Read the model definition and answer for the solid it produces. Units are mm, in the model's axes. Coordinates: 2 decimals unless noted, no trailing zeros. Write each loop counter-clockwise with the first axis right and the second up, starting at its lowest first coordinate (ties: lowest second). Pieces come first, ordered by that corner, then holes.
Item 1: Section B-B (y = 2.85) is taken. Give the vertices of the cut face in (x, z).
Item 2: Section C-C (y = -0.35) is taken. Give the vertices of the cut face in (x, z).
Item 3: Straight lines are drawn through the part: probe 1 along Y at (x, z) = (34.05, 12.5); probe 2 along X at (y, z) = (2.2, 0.25); probe 3 along Y at (x, z) = (35.7, 5.75). For each, find the intervals that lie inside material, in ascending order.
Item 4: Each of these flat-tipped pins is pushed along its axis until it touches: P1, Ø1, axis at x = 33.5, z = -7.5, coming from the +Y side; P2, Ø1.5, axis at x = 34, z = -13, coming from the -Y side; P3, Ø0.9, axis at x = 34.5, y = 0, coming from the -Z side. Where does it stop, or does it pass through?
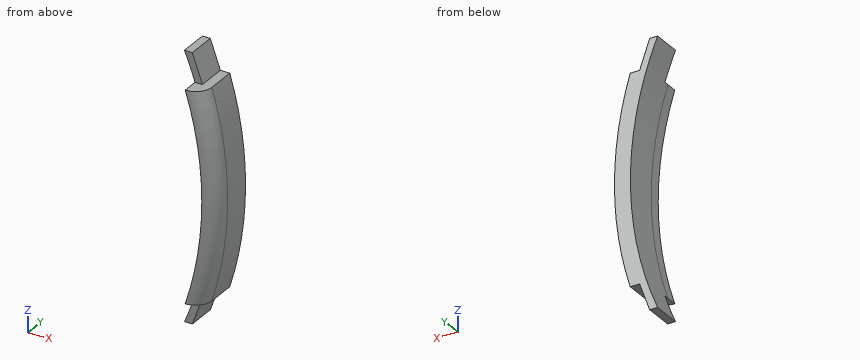
from build123d import *

# Parameters (mm, degrees)
BOSS_EXTRUDE1_DEPTH = 3.6
BOSS_EXTRUDE2_START = 1.2
BOSS_EXTRUDE2_DEPTH = 1.2
FILLET1_R           = 1.7
CUT_EXTRUDE1_DEPTH  = 0.5


with BuildPart() as part:
    # Sketch1 → Boss-Extrude1 (new body)
    with BuildSketch(Plane(origin=(0, 0, 0), x_dir=(1, 0, 0), z_dir=(0, 1, 0))):
        with BuildLine():
            Line((34.819547736, 11.1), (35.819547736, 11.1))
            ThreePointArc((35.819547736, 11.1), (37.5, 0), (35.819547736, -11.1))
            Line((35.819547736, -11.1), (34.819547736, -11.1))
            Line((34.819547736, -11.1), (33.748237365, -14.1))
            Line((33.748237365, -14.1), (32.90638236, -14.1))
            ThreePointArc((32.90638236, -14.1), (35.8, 0), (32.90638236, 14.1))
            Line((32.90638236, 14.1), (33.748237365, 14.1))
            Line((33.748237365, 14.1), (34.819547736, 11.1))
        make_face()
    extrude(amount=BOSS_EXTRUDE1_DEPTH)

    # Sketch2 → Boss-Extrude2 (add)
    with BuildSketch(Plane.XZ.offset(BOSS_EXTRUDE2_START)):
        with BuildLine():
            Line((35.819547736, 11.1), (34.035716534, 11.1))
            ThreePointArc((34.035716534, 11.1), (35.8, 0), (34.035716534, -11.1))
            Line((34.035716534, -11.1), (35.819547736, -11.1))
            ThreePointArc((35.819547736, -11.1), (37.5, 0), (35.819547736, 11.1))
        make_face()
    extrude(amount=-BOSS_EXTRUDE2_DEPTH)

    # Fillet1
    fillet1_edges = [part.edges().sort_by_distance(p)[0] for p in [
        (37.5, -1.2, 0),
    ]]
    fillet(fillet1_edges, radius=FILLET1_R - 0.0001)  # a hair under: the kernel refuses the full size

    # Sketch5 → Cut-Extrude1 (cut)
    with BuildSketch(Plane.XZ):
        with BuildLine():
            Line((34.819547736, -11.1), (34.035716534, -11.1))
            ThreePointArc((34.035716534, -11.1), (33.504643724, -12.612646388), (32.90638236, -14.1))
            Line((32.90638236, -14.1), (33.748237365, -14.1))
            Line((33.748237365, -14.1), (34.819547736, -11.1))
        make_face()
        with BuildLine():
            Line((34.035716534, 11.1), (34.819547736, 11.1))
            Line((34.819547736, 11.1), (33.748237365, 14.1))
            Line((33.748237365, 14.1), (32.90638236, 14.1))
            ThreePointArc((32.90638236, 14.1), (33.504643724, 12.612646388), (34.035716534, 11.1))
        make_face()
    extrude(amount=-CUT_EXTRUDE1_DEPTH, mode=Mode.SUBTRACT)


solid = part.part
Established:
1. outline: (32.91, -14.1) - (33.75, -14.1) - (34.82, -11.1) - (35.82, -11.1) arc R37.5 ccw to (35.82, 11.1) - (34.82, 11.1) - (33.75, 14.1) - (32.91, 14.1) arc R35.8 cw to start
2. outline: (34.04, -11.1) - (35.58, -11.1) arc R37.27 ccw to (35.58, 11.1) - (34.04, 11.1) arc R35.8 cw to start
3. probe 1: y = 0.5 to 3.6
3. probe 2: x = 35.8 to 37.5
3. probe 3: y = -1.16 to 3.6
4. P1: passes through
4. P2: stops at y = 0.5
4. P3: stops at z = -11.1
